Geometry: see drawing. Coordinates: mm, zero at the bounding-box minimum. A direction names the side the tool comes from. Coordinates: 2 decimals unless noted, no trailing zeros. Order: outer loops, then holes, each group sorted by start corner. A loop starts at its lowest first (then second) coordinate and runs counter-clockwise, first axis right, second up. Notation, with made-up numbers: (-18.5, 13.25) -> (-11.5, 13.25) arc R24 cw to (-11.5, 43.25) -> close; hole circle Ø8 at (-21.5, 5). An arc over 180 degrees is marked (long way). Use one line per item in the form item = value.
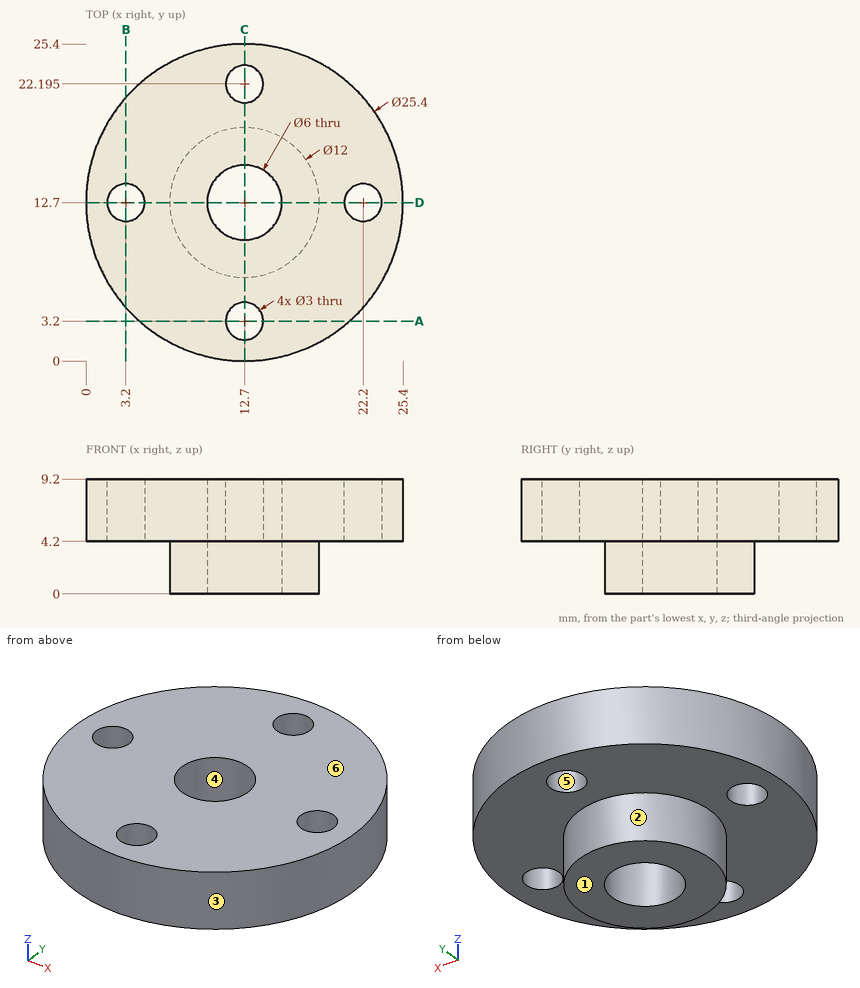
1) Contact query for flat-ended pins moving along their axis: P1, Ø1.5, axis at x = 14.5, z = 3.5, coming from the -Y side; P2, Ø4, axis at x = 14.5, z = 3, coming from the -Y side; P3, Ø1, axis at y = 17.5, z = 5.5, coming from the -X side. Output: stop coordinate, or through.
Results found:
P1 = 0.09
P2 = 0
P3 = 0.75
2) Section A-A, the plane y = 3.2. Output: boundary loops of the cut face in (x, z), and give its area (3 significant figures).
Results found:
outline = (4.27, 4.2) -> (11.2, 4.2) -> (11.2, 9.2) -> (4.27, 9.2) -> close; (14.2, 4.2) -> (21.13, 4.2) -> (21.13, 9.2) -> (14.2, 9.2) -> close
area = 69.3 mm2
3) Pull-direction query (X, two-part tool) for the marked faces 3, 4, 5 and 6; classes: released by +X, released by -X, zero draft, split by the parting line, or undercut.
Results found:
face_3 = split by the parting line
face_4 = undercut
face_5 = undercut
face_6 = zero draft
4) Section C-C, the plane x = 12.7. Output: boundary loops of the cut face in (y, z) (3 decimals).
Results found:
outline = (0, 4.2) -> (1.7, 4.2) -> (1.7, 9.2) -> (0, 9.2) -> close; (4.7, 4.2) -> (6.7, 4.2) -> (6.7, 0) -> (9.7, 0) -> (9.7, 9.2) -> (4.7, 9.2) -> close; (15.7, 0) -> (18.7, 0) -> (18.7, 4.2) -> (20.695, 4.2) -> (20.695, 9.2) -> (15.7, 9.2) -> close; (23.695, 4.2) -> (25.4, 4.2) -> (25.4, 9.2) -> (23.695, 9.2) -> close
5) Access query for the marked faces 1 and 2. Directions: +Z, -Z, +X, -X, +Y, -Y. A direction counts if a zero-diameter tool reaches every point of the face in a straight line with its end or side. Return the directions, or none.
Results found:
face_1 = -Z, +X, -X, +Y, -Y
face_2 = -Z
6) Material intervals for probe 1 along Y at (x, z) = (12.7, 7.3) (3 decimals); probe 2 along X at (y, z) = (11.75, 5) (1 decimal); probe 3 along Y at (x, z) = (15.25, 2), sorted ascending. Write a range as from..to.
Results found:
probe_1 = 0..1.7, 4.7..9.7, 15.7..20.695, 23.695..25.4
probe_2 = 0..2, 4.4..9.9, 15.5..21, 23.4..25.4
probe_3 = 7.27..11.12, 14.28..18.13
7) Section D-D, the plane y = 12.7. Output: boundary loops of the cut face in (x, z).
Results found:
outline = (0, 4.2) -> (1.7, 4.2) -> (1.7, 9.2) -> (0, 9.2) -> close; (4.7, 4.2) -> (6.7, 4.2) -> (6.7, 0) -> (9.7, 0) -> (9.7, 9.2) -> (4.7, 9.2) -> close; (15.7, 0) -> (18.7, 0) -> (18.7, 4.2) -> (20.7, 4.2) -> (20.7, 9.2) -> (15.7, 9.2) -> close; (23.7, 4.2) -> (25.4, 4.2) -> (25.4, 9.2) -> (23.7, 9.2) -> close
